The model under review builds one solid part; all positions refer to its coordinate system, in mm. Face numbers are marked on the shaded views. Give positions to 0.01 mm unless a question says otherwise; leave off trailing zeros. Loops run counter-clockwise (first coordinate to the right, second up) from the corner with the lowest first, then second, coordinate; pieces in that order, holes last. Notation, with made-up numbers: (-3, 50.5) - (26, 50.5) arc R25 cw to (26, 84.5) - close; hole circle Ø7 at (-3, 33). An arc over 180 degrees is marked (long way). Answer as a JSON object with one key per item and string values.
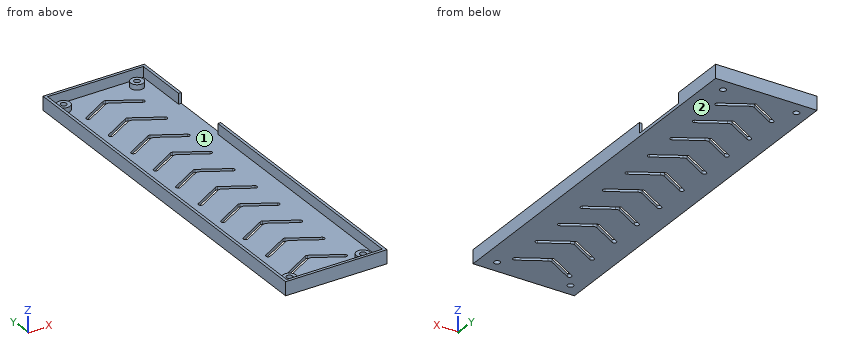
from build123d import *

# Parameters (mm, degrees)
F0_R     = 3.7
F0_W     = 1.6
F0_H     = 35
F1_DEPTH = 1.8
F0_R_2   = 1.7
F2_DEPTH = 4.8
F3_DEPTH = 7.8


with BuildPart() as f1:
    # F0 (on Top) → F1 (new body)
    with BuildSketch(Plane.XY):
        Polygon((56.4, -68), (56.4, -33), (56.4, -1.6), (1.6, -1.6), (1.6, -214.4), (56.4, -214.4), align=None)
        with Locations((7, -208.5)):
            Circle(F0_R, mode=Mode.SUBTRACT)
        with BuildLine():
            Line((11.811543, -199.96077), (27.4, -190.96077))
            ThreePointArc((27.4, -190.96077), (28, -190.8), (28.6, -190.96077))
            Line((28.6, -190.96077), (44.188457, -199.96077))
            ThreePointArc((44.188457, -199.96077), (44.627688, -201.6), (42.988457, -202.03923))
            Line((42.988457, -202.03923), (29.2, -194.078461))
            ThreePointArc((29.2, -194.078461), (28, -193.756922), (26.8, -194.078461))
            Line((26.8, -194.078461), (13.011543, -202.03923))
            ThreePointArc((13.011543, -202.03923), (11.372312, -201.6), (11.811543, -199.96077))
        make_face(mode=Mode.SUBTRACT)
        with BuildLine():
            Line((11.811543, -179.96077), (27.4, -170.96077))
            ThreePointArc((27.4, -170.96077), (28, -170.8), (28.6, -170.96077))
            Line((28.6, -170.96077), (44.188457, -179.96077))
            ThreePointArc((44.188457, -179.96077), (44.627688, -181.6), (42.988457, -182.03923))
            Line((42.988457, -182.03923), (29.2, -174.078461))
            ThreePointArc((29.2, -174.078461), (28, -173.756922), (26.8, -174.078461))
            Line((26.8, -174.078461), (13.011543, -182.03923))
            ThreePointArc((13.011543, -182.03923), (11.372312, -181.6), (11.811543, -179.96077))
        make_face(mode=Mode.SUBTRACT)
        with BuildLine():
            Line((11.811543, -159.96077), (27.4, -150.96077))
            ThreePointArc((27.4, -150.96077), (28, -150.8), (28.6, -150.96077))
            Line((28.6, -150.96077), (44.188457, -159.96077))
            ThreePointArc((44.188457, -159.96077), (44.627688, -161.6), (42.988457, -162.03923))
            Line((42.988457, -162.03923), (29.2, -154.078461))
            ThreePointArc((29.2, -154.078461), (28, -153.756922), (26.8, -154.078461))
            Line((26.8, -154.078461), (13.011543, -162.03923))
            ThreePointArc((13.011543, -162.03923), (11.372312, -161.6), (11.811543, -159.96077))
        make_face(mode=Mode.SUBTRACT)
        with BuildLine():
            Line((11.811543, -139.96077), (27.4, -130.96077))
            ThreePointArc((27.4, -130.96077), (28, -130.8), (28.6, -130.96077))
            Line((28.6, -130.96077), (44.188457, -139.96077))
            ThreePointArc((44.188457, -139.96077), (44.627688, -141.6), (42.988457, -142.03923))
            Line((42.988457, -142.03923), (29.2, -134.078461))
            ThreePointArc((29.2, -134.078461), (28, -133.756922), (26.8, -134.078461))
            Line((26.8, -134.078461), (13.011543, -142.03923))
            ThreePointArc((13.011543, -142.03923), (11.372312, -141.6), (11.811543, -139.96077))
        make_face(mode=Mode.SUBTRACT)
        with BuildLine():
            Line((11.811543, -119.96077), (27.4, -110.96077))
            ThreePointArc((27.4, -110.96077), (28, -110.8), (28.6, -110.96077))
            Line((28.6, -110.96077), (44.188457, -119.96077))
            ThreePointArc((44.188457, -119.96077), (44.627688, -121.6), (42.988457, -122.03923))
            Line((42.988457, -122.03923), (29.2, -114.078461))
            ThreePointArc((29.2, -114.078461), (28, -113.756922), (26.8, -114.078461))
            Line((26.8, -114.078461), (13.011543, -122.03923))
            ThreePointArc((13.011543, -122.03923), (11.372312, -121.6), (11.811543, -119.96077))
        make_face(mode=Mode.SUBTRACT)
        with Locations((49, -208.5)):
            Circle(F0_R, mode=Mode.SUBTRACT)
        with BuildLine():
            Line((11.811543, -99.96077), (27.4, -90.96077))
            ThreePointArc((27.4, -90.96077), (28, -90.8), (28.6, -90.96077))
            Line((28.6, -90.96077), (44.188457, -99.96077))
            ThreePointArc((44.188457, -99.96077), (44.627688, -101.6), (42.988457, -102.03923))
            Line((42.988457, -102.03923), (29.2, -94.078461))
            ThreePointArc((29.2, -94.078461), (28, -93.756922), (26.8, -94.078461))
            Line((26.8, -94.078461), (13.011543, -102.03923))
            ThreePointArc((13.011543, -102.03923), (11.372312, -101.6), (11.811543, -99.96077))
        make_face(mode=Mode.SUBTRACT)
        with BuildLine():
            Line((11.811543, -79.96077), (27.4, -70.96077))
            ThreePointArc((27.4, -70.96077), (28, -70.8), (28.6, -70.96077))
            Line((28.6, -70.96077), (44.188457, -79.96077))
            ThreePointArc((44.188457, -79.96077), (44.627688, -81.6), (42.988457, -82.03923))
            Line((42.988457, -82.03923), (29.2, -74.078461))
            ThreePointArc((29.2, -74.078461), (28, -73.756922), (26.8, -74.078461))
            Line((26.8, -74.078461), (13.011543, -82.03923))
            ThreePointArc((13.011543, -82.03923), (11.372312, -81.6), (11.811543, -79.96077))
        make_face(mode=Mode.SUBTRACT)
        with BuildLine():
            Line((11.811543, -59.96077), (27.4, -50.96077))
            ThreePointArc((27.4, -50.96077), (28, -50.8), (28.6, -50.96077))
            Line((28.6, -50.96077), (44.188457, -59.96077))
            ThreePointArc((44.188457, -59.96077), (44.627688, -61.6), (42.988457, -62.03923))
            Line((42.988457, -62.03923), (29.2, -54.078461))
            ThreePointArc((29.2, -54.078461), (28, -53.756922), (26.8, -54.078461))
            Line((26.8, -54.078461), (13.011543, -62.03923))
            ThreePointArc((13.011543, -62.03923), (11.372312, -61.6), (11.811543, -59.96077))
        make_face(mode=Mode.SUBTRACT)
        with Locations((7, -7.5)):
            Circle(F0_R, mode=Mode.SUBTRACT)
        with BuildLine():
            Line((11.811543, -39.96077), (27.4, -30.96077))
            ThreePointArc((27.4, -30.96077), (28, -30.8), (28.6, -30.96077))
            Line((28.6, -30.96077), (44.188457, -39.96077))
            ThreePointArc((44.188457, -39.96077), (44.627688, -41.6), (42.988457, -42.03923))
            Line((42.988457, -42.03923), (29.2, -34.078461))
            ThreePointArc((29.2, -34.078461), (28, -33.756922), (26.8, -34.078461))
            Line((26.8, -34.078461), (13.011543, -42.03923))
            ThreePointArc((13.011543, -42.03923), (11.372312, -41.6), (11.811543, -39.96077))
        make_face(mode=Mode.SUBTRACT)
        with BuildLine():
            Line((11.811543, -19.96077), (27.4, -10.96077))
            ThreePointArc((27.4, -10.96077), (28, -10.8), (28.6, -10.96077))
            Line((28.6, -10.96077), (44.188457, -19.96077))
            ThreePointArc((44.188457, -19.96077), (44.627688, -21.6), (42.988457, -22.03923))
            Line((42.988457, -22.03923), (29.2, -14.078461))
            ThreePointArc((29.2, -14.078461), (28, -13.756922), (26.8, -14.078461))
            Line((26.8, -14.078461), (13.011543, -22.03923))
            ThreePointArc((13.011543, -22.03923), (11.372312, -21.6), (11.811543, -19.96077))
        make_face(mode=Mode.SUBTRACT)
        with Locations((49, -7.5)):
            Circle(F0_R, mode=Mode.SUBTRACT)
        with Locations((57.2, -50.5)):
            Rectangle(F0_W, F0_H)
    extrude(amount=F1_DEPTH)

    # F0 (on Top) → F2 (join)
    with BuildSketch(Plane.XY):
        with Locations((7, -7.5)):
            Circle(F0_R)
        with Locations((7, -7.5)):
            Circle(F0_R_2, mode=Mode.SUBTRACT)
        with Locations((49, -7.5)):
            Circle(F0_R)
        with Locations((49, -7.5)):
            Circle(F0_R_2, mode=Mode.SUBTRACT)
        with Locations((49, -208.5)):
            Circle(F0_R)
        with Locations((49, -208.5)):
            Circle(F0_R_2, mode=Mode.SUBTRACT)
        with Locations((7, -208.5)):
            Circle(F0_R)
        with Locations((7, -208.5)):
            Circle(F0_R_2, mode=Mode.SUBTRACT)
    extrude(amount=F2_DEPTH)

    # F0 (on Top) → F3 (join)
    with BuildSketch(Plane.XY):
        Polygon((58, 0), (0, 0), (0, -216), (58, -216), (58, -68), (56.4, -68), (56.4, -214.4), (1.6, -214.4), (1.6, -1.6), (56.4, -1.6), (56.4, -33), (58, -33), align=None)
    extrude(amount=F3_DEPTH)


solid = f1.part
Q1. The part is to be moulded in two halves that separate along Y. For the marked faces 1 and 2, say which applies: +Y half, -Y half, draft (parallel to the pull), parting line (faces both ways), or undercut.
Results:
{"face 1": "undercut", "face 2": "draft"}
Q2. Clearance check with flat-ended pins moving along their axes: pin 1 Ø5 at (x, y) = (27.5, -148) entering from -Z; pin 2 Ø2 at (x, y) = (49.5, -8.5) entering from +Z. State where each tip first meets the part, or that it passes through.
Results:
{"pin 1": "stops at z = 0", "pin 2": "stops at z = 4.8"}
Q3. To check wall thickness, follow probe 1 along Y at (x, z) = (7, 1.05); probe 2 along Y at (x, z) = (49, 3.55); probe 3 along X at (y, z) = (-208.5, 3.1). State the ranges of each line that lie inside material, in increasing order. Write a range as [from, to].
Results:
{"probe 1": "y = [-216, -210.2], [-206.8, -9.2], [-5.8, 0]", "probe 2": "y = [-216, -214.4], [-212.2, -210.2], [-206.8, -204.8], [-11.2, -9.2], [-5.8, -3.8], [-1.6, 0]", "probe 3": "x = [0, 1.6], [3.3, 5.3], [8.7, 10.7], [45.3, 47.3], [50.7, 52.7], [56.4, 58]"}
Q4. Consider section B-B, the plane y = -66. State the section outline as (x, z) points, plus the area to 3 significant figures.
Results:
{"outline": "(0, 0) - (58, 0) - (58, 1.8) - (1.6, 1.8) - (1.6, 7.8) - (0, 7.8) - close", "area": "114 mm^2"}
Q5. Consider section A-A, the plane z = 3.5. State how many separate pieces and enclosed holes the cut face has, plus the area to 3 significant figures.
Results:
{"separate pieces": "5", "enclosed holes": "4", "area": "946 mm^2"}
